Can you work these out from the model? Positions are in its coordinate system, mm. A direction names the side the tool comes from. Give positions to 0.01 mm unless a question says otherwise; leave off trailing zeros. Write each loop counter-clockwise with the first axis right and the second up, starting at its lowest first coordinate (ties: lowest second). Pieces come first, ordered by that corner, then holes. Notation, with made-up numbers: (-8, 80) -> (19, 80) arc R20 cw to (19, 95) -> close; hole circle Ø2 at (88, 38.25). An arc over 180 degrees is marked (long way). Answer as CSV lines item,"result". Start each with the question number.
1. If we section it at A-A on x = 193: Write out the boundary of the cut face in (y, z), plus the area to 3 significant figures.
2. On a 3-axis mill with a long thin cutter (end or side, diameter ignored), from which of +Z, -Z, +X, -X, +Y, -Y can I reach the whole of each face in a straight line? I mean faces 3 (the face through (96.62, 68.53, 6.26)), 4 (the face through (117.28, 39, 6)), 5 (the face through (147, 6.35, 120)), 6 (the face through (108, 88.9, 5)). Say none if no direction works.
3. I'm going to push flat-ended pins straight in: P1, Ø14, axis at y = 7.5, z = 79.5, coming from the -X side; P2, Ø10, axis at y = 124, z = 142.5, coming from the +X side; P3, Ø6.5, axis at y = 82.5, z = 8, coming from the -X side; P4, Ø4, axis at x = 187.5, z = 160, coming from the +Y side. Where does each tip first touch, or does it pass through?
4. If we section it at B-B on y = 61: Write out the boundary of the cut face in (x, z).
5. If we mould it in two halves opening along Z, with no side actions, what happens to faces 1 (the face through (215.705, 6, 159)), 2 (the face through (67, 10, 12.7))? For each: pulls with the +Z half, pulls with the -Z half, needs draft (parallel to the pull), parting line crosses it, or undercut.
6. I need wall thicknesses on line 1 (X direction, y = 133, z = 9.5); line 2 (Y direction, x = 175, z = 146.5). Which ranges of each line are inside material? Lowest first, please. Write a range as [from, to].
```python
from build123d import *

# Parameters (mm, degrees)
BOSS_EXTRUDE2_DEPTH  = 6.35
BOSS_EXTRUDE3_DEPTH  = 6.35
SKETCH3_W            = 1.5875
SKETCH3_H            = 158.75
BOSS_EXTRUDE4_DEPTH  = 6.35
SKETCH4_W            = 12.7
SKETCH4_H            = 6.35
BOSS_EXTRUDE5_DEPTH  = 158.75
SKETCH5_W            = 12.7
SKETCH5_H            = 6.35
BOSS_EXTRUDE6_DEPTH  = 158.75
SKETCH6_W            = 1.5875
SKETCH6_H            = 158.75
BOSS_EXTRUDE7_DEPTH  = 6.35
SKETCH7_W            = 1.5875
SKETCH7_H            = 158.75
BOSS_EXTRUDE8_DEPTH  = 6.35
SKETCH8_W            = 1.5875
SKETCH8_H            = 6.35
BOSS_EXTRUDE9_DEPTH  = 139.7
SKETCH10_W           = 1.5875
SKETCH10_H           = 6.35
BOSS_EXTRUDE10_DEPTH = 139.7
SKETCH11_W           = 12.7
SKETCH11_H           = 12.699759929
BOSS_EXTRUDE11_DEPTH = 101.6
SKETCH12_W           = 101.404934815
SKETCH12_H           = 12.7
BOSS_EXTRUDE12_DEPTH = 6.35
SKETCH13_W           = 101.6
SKETCH13_H           = 12.7
BOSS_EXTRUDE13_DEPTH = 6.35
SKETCH14_W           = 12.7
SKETCH14_H           = 12.7
BOSS_EXTRUDE14_DEPTH = 101.6
SKETCH15_W           = 139.7
SKETCH15_H           = 6.35
BOSS_EXTRUDE15_DEPTH = 63.5
CUT_EXTRUDE1_DEPTH   = 3.175
CUT_EXTRUDE1_DRAFT   = 15
CUT_EXTRUDE3_DEPTH   = 6.35
SKETCH18_W           = 12.7
SKETCH18_H           = 152.4
BOSS_EXTRUDE17_DEPTH = 3.175
SKETCH19_W           = 12.7
SKETCH19_H           = 152.4
BOSS_EXTRUDE18_DEPTH = 3.175
SKETCH20_W           = 12.7
SKETCH20_H           = 152.4
BOSS_EXTRUDE19_DEPTH = 3.175
SKETCH21_W           = 12.7
SKETCH21_H           = 152.4
BOSS_EXTRUDE20_DEPTH = 3.175
SKETCH22_W           = 139.7
SKETCH22_H           = 6.35
BOSS_EXTRUDE21_DEPTH = 3.175
SKETCH23_W           = 139.7
SKETCH23_H           = 12.699759929
BOSS_EXTRUDE22_DEPTH = 3.175
CUT_EXTRUDE4_DEPTH   = 12.7
SKETCH30_W           = 12.7
SKETCH30_H           = 26.035
BOSS_EXTRUDE25_DEPTH = 3.175
SKETCH31_W           = 12.7
SKETCH31_H           = 26.035
BOSS_EXTRUDE26_DEPTH = 3.175
BOSS_EXTRUDE27_DEPTH = 12.7
BOSS_EXTRUDE28_DEPTH = 12.7
SKETCH37_R           = 0.635
BOSS_EXTRUDE29_DEPTH = 7.9375


with BuildPart() as part:
    # Sketch1 → Boss-Extrude2 (new body)
    with BuildSketch(Plane.XY):
        Polygon((0, 0), (215.704934815, 0), (215.704934815, 12.7), (114.104934815, 12.7), (114.104934815, 165.1), (101.404934815, 165.1), (101.404934815, 12.7), (0, 12.7), align=None)
    extrude(amount=BOSS_EXTRUDE2_DEPTH)

    # Sketch2 → Boss-Extrude3 (add)
    with BuildSketch(Plane.XY.offset(6.35)):
        Polygon((101.404934815, 12.7), (101.404934815, 6.35), (102.992434815, 6.35), (102.992434815, 165.1), (101.404934815, 165.1), align=None)
    extrude(amount=BOSS_EXTRUDE3_DEPTH)

    # Sketch3 → Boss-Extrude4 (add)
    with BuildSketch(Plane.XY.offset(6.35)):
        with Locations((113.311184815, 85.725)):
            Rectangle(SKETCH3_W, SKETCH3_H)
    extrude(amount=BOSS_EXTRUDE4_DEPTH)

    # Sketch4 → Boss-Extrude5 (add)
    with BuildSketch(Plane.XY.offset(6.35)):
        with Locations((107.754934815, 3.175)):
            Rectangle(SKETCH4_W, SKETCH4_H)
    extrude(amount=BOSS_EXTRUDE5_DEPTH)

    # Sketch5 → Boss-Extrude6 (add)
    with BuildSketch(Plane(origin=(0, 6.35, 0), x_dir=(1, 0, 0), z_dir=(0, 1, 0))):
        with Locations((107.754934815, -161.925)):
            Rectangle(SKETCH5_W, SKETCH5_H)
    extrude(amount=BOSS_EXTRUDE6_DEPTH)

    # Sketch6 → Boss-Extrude7 (add)
    with BuildSketch(Plane(origin=(0, 0, 158.75), x_dir=(-1, 0, 0), z_dir=(0, 0, -1))):
        with Locations((-102.198684815, 85.725)):
            Rectangle(SKETCH6_W, SKETCH6_H)
    extrude(amount=BOSS_EXTRUDE7_DEPTH)

    # Sketch7 → Boss-Extrude8 (add)
    with BuildSketch(Plane(origin=(0, 0, 158.75), x_dir=(-1, 0, 0), z_dir=(0, 0, -1))):
        with Locations((-113.311184815, 85.725)):
            Rectangle(SKETCH7_W, SKETCH7_H)
    extrude(amount=BOSS_EXTRUDE8_DEPTH)

    # Sketch8 → Boss-Extrude9 (add)
    with BuildSketch(Plane(origin=(0, 0, 152.4), x_dir=(-1, 0, 0), z_dir=(0, 0, -1))):
        with Locations((-113.311184815, 9.525)):
            Rectangle(SKETCH8_W, SKETCH8_H)
    extrude(amount=BOSS_EXTRUDE9_DEPTH)

    # Sketch10 → Boss-Extrude10 (add)
    with BuildSketch(Plane.XY.offset(12.7)):
        with Locations((102.198684815, 9.525)):
            Rectangle(SKETCH10_W, SKETCH10_H)
    extrude(amount=BOSS_EXTRUDE10_DEPTH)

    # Sketch11 → Boss-Extrude11 (add)
    with BuildSketch(Plane.ZY.offset(-101.404934815)):
        with Locations((158.75, 6.349879965)):
            Rectangle(SKETCH11_W, SKETCH11_H)
    extrude(amount=BOSS_EXTRUDE11_DEPTH)

    # Sketch12 → Boss-Extrude12 (add)
    with BuildSketch(Plane.XY.offset(6.35)):
        with Locations((50.702467408, 6.35)):
            Rectangle(SKETCH12_W, SKETCH12_H)
    extrude(amount=BOSS_EXTRUDE12_DEPTH)

    # Sketch13 → Boss-Extrude13 (add)
    with BuildSketch(Plane.XY.offset(6.35)):
        with Locations((164.904934815, 6.35)):
            Rectangle(SKETCH13_W, SKETCH13_H)
    extrude(amount=BOSS_EXTRUDE13_DEPTH)

    # Sketch14 → Boss-Extrude14 (add)
    with BuildSketch(Plane(origin=(114.104934815, 0, 0), x_dir=(0, 0, -1), z_dir=(1, 0, 0))):
        with Locations((-158.75, 6.35)):
            Rectangle(SKETCH14_W, SKETCH14_H)
    extrude(amount=BOSS_EXTRUDE14_DEPTH)

    # Sketch15 → Boss-Extrude15 (add)
    with BuildSketch(Plane(origin=(114.104934815, 0, 0), x_dir=(0, 0, -1), z_dir=(1, 0, 0))):
        with Locations((-82.55, 3.175)):
            Rectangle(SKETCH15_W, SKETCH15_H)
    extrude(amount=BOSS_EXTRUDE15_DEPTH)


with BuildPart() as cut_extrude1_tool:
    # Sketch16 → Cut-Extrude1 (with draft: the straight prism first)
    with BuildSketch(Plane(origin=(0, 6.35, 0), x_dir=(1, 0, 0), z_dir=(0, 1, 0))):
        Polygon((177.604934815, -82.55), (177.604934815, -79.375), (114.104934815, -79.375), (114.104934815, -82.55), (114.104934815, -85.725), (177.604934815, -85.725), align=None)
    extrude(amount=-CUT_EXTRUDE1_DEPTH)
    # Cut-Extrude1: the draft: its side faces are tilted about the plane it starts from
    cut_extrude1_sides = [cut_extrude1_tool.faces().sort_by_distance(p)[0] for p in [
        (177.604934815, 4.7625, 82.55),
        (114.104934815, 4.7625, 82.55),
        (145.854934815, 4.7625, 85.725),
        (145.854934815, 4.7625, 79.375),
    ]]
    draft(cut_extrude1_sides, Plane(origin=(0, 6.35, 0), x_dir=(1, 0, 0), z_dir=(0, 1, 0)), CUT_EXTRUDE1_DRAFT)


with BuildPart() as part_1:
    add(part.part)

    # Cut-Extrude1: cut by cut_extrude1_tool
    add(cut_extrude1_tool.part, mode=Mode.SUBTRACT)

    # Sketch17 → Cut-Extrude3 (cut)
    with BuildSketch(Plane(origin=(0, 0, 0), x_dir=(-1, 0, 0), z_dir=(0, 0, -1))):
        Polygon((-107.803701111, 87.3125), (-112.566201111, 87.3125), (-112.566201111, 82.55), (-112.566201111, 77.784684897), (-107.806516214, 77.784684897), (-103.041201111, 77.784684897), (-103.041201111, 82.55), (-103.041201111, 87.3125), align=None)
    extrude(amount=-CUT_EXTRUDE3_DEPTH, mode=Mode.SUBTRACT)

    # Sketch18 → Boss-Extrude17 (add)
    with BuildSketch(Plane.ZY.offset(-101.404934815)):
        with Locations((6.35, 88.9)):
            Rectangle(SKETCH18_W, SKETCH18_H)
    extrude(amount=BOSS_EXTRUDE17_DEPTH)

    # Sketch19 → Boss-Extrude18 (add)
    with BuildSketch(Plane(origin=(114.104934815, 0, 0), x_dir=(0, 0, -1), z_dir=(1, 0, 0))):
        with Locations((-6.35, 88.9)):
            Rectangle(SKETCH19_W, SKETCH19_H)
    extrude(amount=BOSS_EXTRUDE18_DEPTH)

    # Sketch20 → Boss-Extrude19 (add)
    with BuildSketch(Plane.ZY.offset(-101.404934815)):
        with Locations((158.75, 88.9)):
            Rectangle(SKETCH20_W, SKETCH20_H)
    extrude(amount=BOSS_EXTRUDE19_DEPTH)

    # Sketch21 → Boss-Extrude20 (add)
    with BuildSketch(Plane(origin=(114.104934815, 0, 0), x_dir=(0, 0, -1), z_dir=(1, 0, 0))):
        with Locations((-158.75, 88.9)):
            Rectangle(SKETCH21_W, SKETCH21_H)
    extrude(amount=BOSS_EXTRUDE20_DEPTH)

    # Sketch22 → Boss-Extrude21 (add)
    with BuildSketch(Plane(origin=(114.104934815, 0, 0), x_dir=(0, 0, -1), z_dir=(1, 0, 0))):
        with Locations((-82.55, 9.525)):
            Rectangle(SKETCH22_W, SKETCH22_H)
    extrude(amount=BOSS_EXTRUDE21_DEPTH)

    # Sketch23 → Boss-Extrude22 (add)
    with BuildSketch(Plane.ZY.offset(-101.404934815)):
        with Locations((82.55, 6.349879965)):
            Rectangle(SKETCH23_W, SKETCH23_H)
    extrude(amount=BOSS_EXTRUDE22_DEPTH)

    # Sketch25 → Cut-Extrude4 (cut)
    with BuildSketch(Plane(origin=(0, 0, 0), x_dir=(-1, 0, 0), z_dir=(0, 0, -1))):
        Polygon((-112.566201111, 88.9), (-101.453701111, 88.9), (-101.453701111, 76.2), (-114.153701111, 76.2), (-114.153701111, 88.9), align=None)
    extrude(amount=-CUT_EXTRUDE4_DEPTH, mode=Mode.SUBTRACT)

    # Sketch30 → Boss-Extrude25 (add)
    with BuildSketch(Plane(origin=(117.279934815, 0, 0), x_dir=(0, 0, -1), z_dir=(1, 0, 0))):
        with Locations((-6.35, 86.0425)):
            Rectangle(SKETCH30_W, SKETCH30_H)
    extrude(amount=BOSS_EXTRUDE25_DEPTH)

    # Sketch31 → Boss-Extrude26 (add)
    with BuildSketch(Plane.ZY.offset(-98.229934815)):
        with Locations((6.35, 86.0425)):
            Rectangle(SKETCH31_W, SKETCH31_H)
    extrude(amount=BOSS_EXTRUDE26_DEPTH)

    # Sketch32 → Boss-Extrude27 (add)
    with BuildSketch(Plane(origin=(0, 0, 0), x_dir=(-1, 0, 0), z_dir=(0, 0, -1))):
        Polygon((-120.454934815, 73.025), (-117.279934815, 63.840058945), (-117.279934815, 73.025), align=None)
    extrude(amount=-BOSS_EXTRUDE27_DEPTH)

    # Sketch36 → Boss-Extrude28 (add)
    with BuildSketch(Plane(origin=(0, 0, 0), x_dir=(-1, 0, 0), z_dir=(0, 0, -1))):
        Polygon((-95.054934815, 73.025), (-98.229934815, 63.911198594), (-98.229934815, 73.025), align=None)
    extrude(amount=-BOSS_EXTRUDE28_DEPTH)

    # Sketch37 → Boss-Extrude29 (add)
    with BuildSketch(Plane(origin=(0, 0, 0), x_dir=(-1, 0, 0), z_dir=(0, 0, -1))):
        with Locations(Location((-117.803681111, 82.55, 0), (0, 0, 180))):
            Circle(SKETCH37_R)
        with Locations(Location((-96.803672311, 82.55, 0), (0, 0, 180))):
            Circle(SKETCH37_R)
        with Locations(Location((-96.803672311, 94.5500014, 0), (0, 0, 180))):
            Circle(SKETCH37_R)
        with Locations(Location((-117.803681111, 94.5500014, 0), (0, 0, 180))):
            Circle(SKETCH37_R)
    extrude(amount=BOSS_EXTRUDE29_DEPTH)


solid = part_1.part
```
Computed values:
1,outline,"(0, 0) -> (12.7, 0) -> (12.7, 12.7) -> (0, 12.7) -> close; (0, 152.4) -> (12.7, 152.4) -> (12.7, 165.1) -> (0, 165.1) -> close"
1,area,"323 mm2"
2,face 3,"+Z, -Z, -X"
2,face 4,"+Z, -Z, +X"
2,face 5,"+X, +Y"
2,face 6,"-Z"
3,P1,"stops at x = 98.23"
3,P2,"passes through"
3,P3,"stops at x = 95.05"
3,P4,"stops at y = 12.7"
4,outline,"(98.23, 0) -> (117.28, 0) -> (117.28, 12.7) -> (112.52, 12.7) -> (112.52, 6.35) -> (102.99, 6.35) -> (102.99, 12.7) -> (98.23, 12.7) -> close; (98.23, 152.4) -> (102.99, 152.4) -> (102.99, 158.75) -> (112.52, 158.75) -> (112.52, 152.4) -> (117.28, 152.4) -> (117.28, 165.1) -> (98.23, 165.1) -> close"
5,face 1,"needs draft"
5,face 2,"undercut"
6,line 1,"x = [98.23, 102.99], [112.52, 117.28]"
6,line 2,"y = [0, 6.35]"
